Geometry check sheet. Reference: the model listing, model coordinates, mm. Face numbers are marked on the shaded views. Coordinates: 2 decimals unless noted, no trailing zeros. Loops run counter-clockwise (first coordinate to the right, second up) from the corner with the lowest first, then second, coordinate; pieces in that order, holes last. Notation, with made-up numbers: (87.25, 67.25) - (146.25, 67.25) arc R19 cw to (146.25, 104.25) - close; hole circle Ø1 at (29, 36). An arc over 180 degrees is marked (long way). Write item = value, one per line. Start each with the question number.
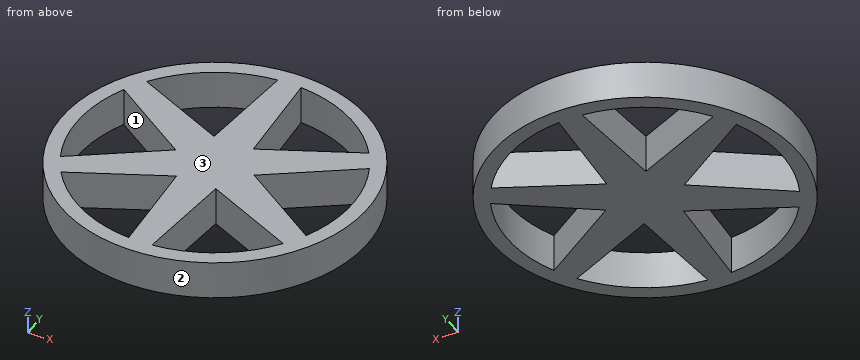
from build123d import *

# Parameters (mm, degrees)
F0_R     = 20
F1_DEPTH = 5


with BuildPart() as f1:
    # F0 (on Top) → F1 (new body)
    with BuildSketch(Plane.XY):
        Circle(F0_R)
        with BuildLine():
            Line((-14.757616, -10.305958), (-2.605141, -4.512237))
            Line((-2.605141, -4.512237), (-1.546413, -17.933449))
            ThreePointArc((-1.546413, -17.933449), (-9, -15.588457), (-14.757616, -10.305958))
        make_face(mode=Mode.SUBTRACT)
        with BuildLine():
            Line((1.546413, -17.933449), (2.605141, -4.512237))
            Line((2.605141, -4.512237), (14.757616, -10.305958))
            ThreePointArc((14.757616, -10.305958), (9, -15.588457), (1.546413, -17.933449))
        make_face(mode=Mode.SUBTRACT)
        with BuildLine():
            Line((16.304029, -7.627492), (5.210282, 0))
            Line((5.210282, 0), (16.304029, 7.627492))
            ThreePointArc((16.304029, 7.627492), (18, 0), (16.304029, -7.627492))
        make_face(mode=Mode.SUBTRACT)
        with BuildLine():
            Line((-16.304029, 7.627492), (-5.210282, 0))
            Line((-5.210282, 0), (-16.304029, -7.627492))
            ThreePointArc((-16.304029, -7.627492), (-18, 0), (-16.304029, 7.627492))
        make_face(mode=Mode.SUBTRACT)
        with BuildLine():
            ThreePointArc((-14.757616, 10.305958), (-9, 15.588457), (-1.546413, 17.933449))
            Line((-1.546413, 17.933449), (-2.605141, 4.512237))
            Line((-2.605141, 4.512237), (-14.757616, 10.305958))
        make_face(mode=Mode.SUBTRACT)
        with BuildLine():
            Line((14.757616, 10.305958), (2.605141, 4.512237))
            Line((2.605141, 4.512237), (1.546413, 17.933449))
            ThreePointArc((1.546413, 17.933449), (9, 15.588457), (14.757616, 10.305958))
        make_face(mode=Mode.SUBTRACT)
    extrude(amount=F1_DEPTH)


solid = f1.part
(1) Draft check along X on the marked faces 1, 2 and 3. Enter one of: pulls with the +X half, pulls with the -X half, needs draft (parallel to the pull), parting line crosses it, or undercut.
(2) Sectioned sample at C-C on x = 8. Enter the section's corners in (y, z).
(3) Depth check by flat-ended pin: pin 1 (1 mm diameter, centred on x = -5.5, z = 2, fed in from -Y). Enter the tip coordinate at first touch or a pass-through.
(4) Sectioned sample at B-B on x = -12. Enter the section's corners in (y, z), plus the area to 3 significant figures.
(5) Sectioned sample at A-A on z = 3.9. Enter the section's corners in (x, y).
(6) Scan lines: line 1 (Y direction, x = -6, z = 4.45); line 2 (X direction, y = -10, z = 0.7); line 3 (Y direction, x = -10, z = 0.85). Record each from-to range of solid material in increasing order.
Working result:
q1.face_1 = undercut
q1.face_2 = parting line crosses it
q1.face_3 = needs draft
q2.outline = (-18.33, 0) - (-16.12, 0) - (-16.12, 5) - (-18.33, 5) - close; (-7.08, 0) - (-1.92, 0) - (-1.92, 5) - (-7.08, 5) - close; (1.92, 0) - (7.08, 0) - (7.08, 5) - (1.92, 5) - close; (16.12, 0) - (18.33, 0) - (18.33, 5) - (16.12, 5) - close
q3.pin_1 = -19.36
q4.outline = (-16, 0) - (-13.42, 0) - (-13.42, 5) - (-16, 5) - close; (-8.99, 0) - (-4.67, 0) - (-4.67, 5) - (-8.99, 5) - close; (4.67, 0) - (8.99, 0) - (8.99, 5) - (4.67, 5) - close; (13.42, 0) - (16, 0) - (16, 5) - (13.42, 5) - close
q4.area = 69.1 mm2
q5.outline = circle Ø40 at (0, 0); hole (-16.3, -7.63) - (-5.21, 0) - (-16.3, 7.63) arc R18 ccw to start; hole (-14.76, -10.31) arc R18 ccw to (-1.55, -17.93) - (-2.61, -4.51) - close; hole (-14.76, 10.31) - (-2.61, 4.51) - (-1.55, 17.93) arc R18 ccw to start; hole (1.55, -17.93) arc R18 ccw to (14.76, -10.31) - (2.61, -4.51) - close; hole (1.55, 17.93) - (2.61, 4.51) - (14.76, 10.31) arc R18 ccw to start; hole (5.21, 0) - (16.3, -7.63) arc R18 ccw to (16.3, 7.63) - close
q6.line_1 = -19.08 to -16.97, -6.13 to -0.54, 0.54 to 6.13, 16.97 to 19.08
q6.line_2 = -17.32 to -14.12, -2.17 to 2.17, 14.12 to 17.32
q6.line_3 = -17.32 to -14.97, -8.04 to -3.29, 3.29 to 8.04, 14.97 to 17.32
